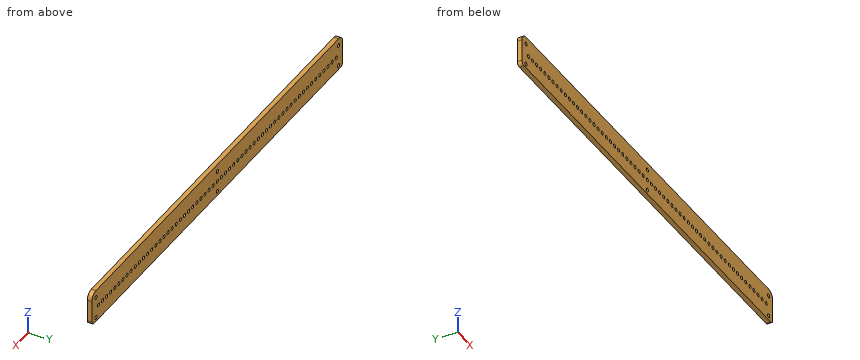
```python
from build123d import *

# Parameters (mm, degrees)
BOSS_EXTRUDE1_DEPTH   = 6.35
M6X1_0_TAPPED_HOLE2_D = 5
LPATTERN2_COUNT       = 59
LPATTERN2_PITCH       = 10
CUT_EXTRUDE1_REACH    = 8.35
SKETCH8_R             = 2.6


with BuildPart() as part:
    # Sketch1 → Boss-Extrude1 (new body)
    with BuildSketch(Plane(origin=(0, 0, 0), x_dir=(1, 0, 0), z_dir=(0, 1, 0))):
        with BuildLine():
            Line((10, 0), (601.6, 0))
            ThreePointArc((601.6, 0), (608.671067812, 2.928932188), (611.6, 10))
            Line((611.6, 10), (611.6, 40))
            ThreePointArc((611.6, 40), (610.135533906, 43.535533906), (606.6, 45))
            Line((606.6, 45), (5, 45))
            ThreePointArc((5, 45), (1.464466094, 43.535533906), (0, 40))
            Line((0, 40), (0, 10))
            ThreePointArc((0, 10), (2.928932188, 2.928932188), (10, 0))
        make_face()
    extrude(amount=BOSS_EXTRUDE1_DEPTH)

    # M6x1.0 Tapped Hole2 (through all)
    with Locations(Plane(origin=(0, 6.35, 0), x_dir=(1, 0, 0), z_dir=(0, 1, 0))):
        with Locations((595.8, 24.6)):
            m6x1_0_tapped_hole2 = Hole(M6X1_0_TAPPED_HOLE2_D / 2)

    # LPattern2: M6x1.0 Tapped Hole2 ×59
    with Locations(*[(-i * LPATTERN2_PITCH, 0, 0) for i in range(1, LPATTERN2_COUNT)]):
        add(m6x1_0_tapped_hole2, mode=Mode.SUBTRACT)

    # Sketch8 → Cut-Extrude1 (cut, up to next)
    with BuildSketch(Plane(origin=(0, 6.35, 0), x_dir=(1, 0, 0), z_dir=(0, 1, 0)), mode=Mode.PRIVATE) as cut_extrude1_sk1:
        with Locations((10, 10)):
            Circle(SKETCH8_R)
    cut_extrude1_tool1 = extrude(cut_extrude1_sk1.sketch, amount=-CUT_EXTRUDE1_REACH, mode=Mode.PRIVATE) & part.part
    add(cut_extrude1_tool1.solids().sort_by_distance((10, 6.35, -10))[0], mode=Mode.SUBTRACT)
    # Sketch8 → Cut-Extrude1 (cut, up to next)
    with BuildSketch(Plane(origin=(0, 6.35, 0), x_dir=(1, 0, 0), z_dir=(0, 1, 0)), mode=Mode.PRIVATE) as cut_extrude1_sk2:
        with Locations((10, 39.2)):
            Circle(SKETCH8_R)
    cut_extrude1_tool2 = extrude(cut_extrude1_sk2.sketch, amount=-CUT_EXTRUDE1_REACH, mode=Mode.PRIVATE) & part.part
    add(cut_extrude1_tool2.solids().sort_by_distance((10, 6.35, -39.2))[0], mode=Mode.SUBTRACT)
    # Sketch8 → Cut-Extrude1 (cut, up to next)
    with BuildSketch(Plane(origin=(0, 6.35, 0), x_dir=(1, 0, 0), z_dir=(0, 1, 0)), mode=Mode.PRIVATE) as cut_extrude1_sk3:
        with Locations((601.6, 10)):
            Circle(SKETCH8_R)
    cut_extrude1_tool3 = extrude(cut_extrude1_sk3.sketch, amount=-CUT_EXTRUDE1_REACH, mode=Mode.PRIVATE) & part.part
    add(cut_extrude1_tool3.solids().sort_by_distance((601.6, 6.35, -10))[0], mode=Mode.SUBTRACT)
    # Sketch8 → Cut-Extrude1 (cut, up to next)
    with BuildSketch(Plane(origin=(0, 6.35, 0), x_dir=(1, 0, 0), z_dir=(0, 1, 0)), mode=Mode.PRIVATE) as cut_extrude1_sk4:
        with Locations((601.6, 39.2)):
            Circle(SKETCH8_R)
    cut_extrude1_tool4 = extrude(cut_extrude1_sk4.sketch, amount=-CUT_EXTRUDE1_REACH, mode=Mode.PRIVATE) & part.part
    add(cut_extrude1_tool4.solids().sort_by_distance((601.6, 6.35, -39.2))[0], mode=Mode.SUBTRACT)
    # Sketch8 → Cut-Extrude1 (cut, up to next)
    with BuildSketch(Plane(origin=(0, 6.35, 0), x_dir=(1, 0, 0), z_dir=(0, 1, 0)), mode=Mode.PRIVATE) as cut_extrude1_sk5:
        with Locations((305.8, 10)):
            Circle(SKETCH8_R)
    cut_extrude1_tool5 = extrude(cut_extrude1_sk5.sketch, amount=-CUT_EXTRUDE1_REACH, mode=Mode.PRIVATE) & part.part
    add(cut_extrude1_tool5.solids().sort_by_distance((305.8, 6.35, -10))[0], mode=Mode.SUBTRACT)
    # Sketch8 → Cut-Extrude1 (cut, up to next)
    with BuildSketch(Plane(origin=(0, 6.35, 0), x_dir=(1, 0, 0), z_dir=(0, 1, 0)), mode=Mode.PRIVATE) as cut_extrude1_sk6:
        with Locations((305.8, 39.2)):
            Circle(SKETCH8_R)
    cut_extrude1_tool6 = extrude(cut_extrude1_sk6.sketch, amount=-CUT_EXTRUDE1_REACH, mode=Mode.PRIVATE) & part.part
    add(cut_extrude1_tool6.solids().sort_by_distance((305.8, 6.35, -39.2))[0], mode=Mode.SUBTRACT)


solid = part.part
```
Geometry check sheet. Reference: the model listing, model coordinates, mm. Give positions to 0.01 mm unless a question says otherwise; leave off trailing zeros.
1. Thickness scan on L1, parallel to X at y = 5, z = -39; L2, parallel to Z at x = 395.8, y = 1.5; L3, parallel to Z at x = 476.5, y = 5.25. Record the ranges inside material, lowest first.
2. Gauge pin test, flat end, axial feed: pin 1 Ø3 at (x, z) = (145.8, -24.6) entering from +Y. Record the tip position at first contact, or that the pin passes through.
3. Section check A-A, the plane y = 4.75. Give the number of separate pieces and of enclosed holes in the cut face, and give its area (3 significant figures).
Values follow:
1. L1: x = 0 to 7.41, 12.59 to 303.21, 308.39 to 599.01, 604.19 to 611.6
1. L2: z = -45 to -27.1, -22.1 to 0
1. L3: z = -45 to -27, -22.2 to 0
2. pin 1: passes through
3. separate pieces: 1
3. enclosed holes: 65
3. area: 26,200 mm2
